Input: dimensioned drawing with shaded views. Units: mm. Origin: part minimum x, y, z. Give positions to 0.01 mm unless a question says otherwise; leave off trailing zeros. Loops run counter-clockwise (first coordinate to the right, second up) from the corner with the lowest first, then second, coordinate; pieces in that order, holes last. Notation, with made-up numbers: (4.25, 8.25) -> (63.25, 8.25) arc R28 cw to (63.25, 28.25) -> close; hole circle Ø3 at (30.25, -5.75). An arc over 180 degrees is marked (long way). Answer as a JSON object with one key per item and string values.
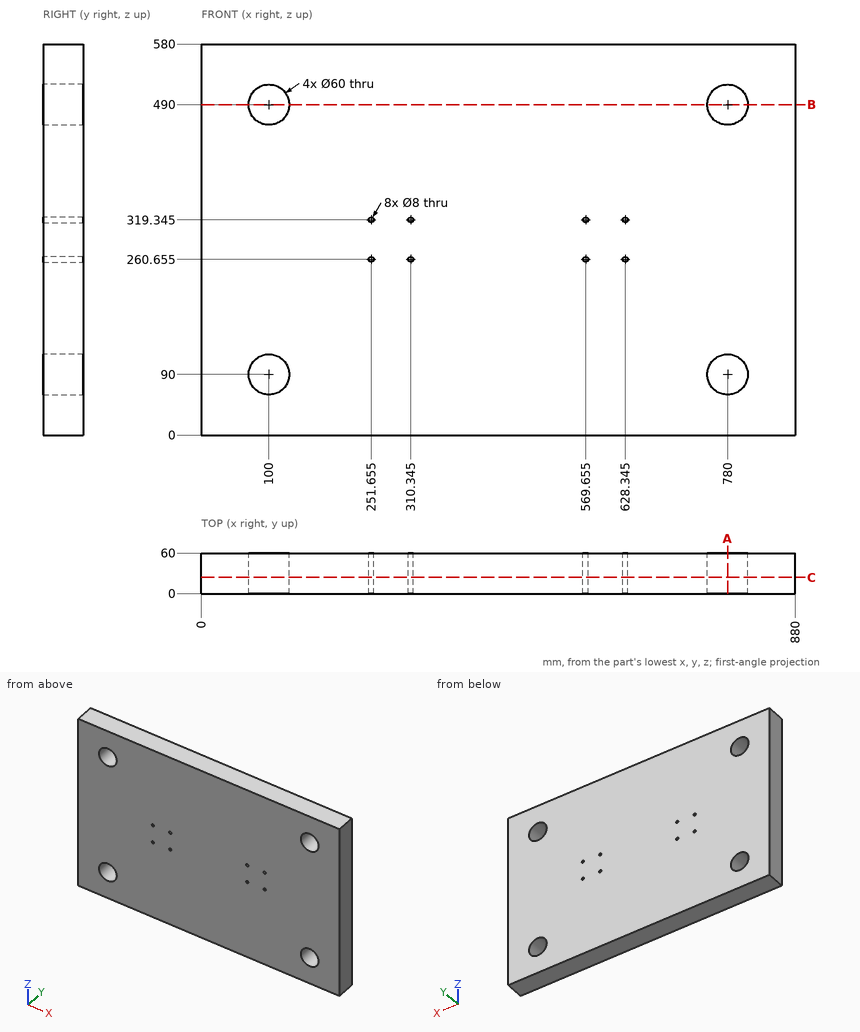
Q1. Ray query, line 1 along X through (y, z) = (57, 261); line 2 along X through (y, z) = (15, 90); line 3 along Z through (x, y) = (254, 46.5). Return the intervals inside material, ascending.
Evaluation:
{"line 1": "x = 0 to 247.67, 255.64 to 306.36, 314.33 to 565.67, 573.64 to 624.36, 632.33 to 880", "line 2": "x = 0 to 70, 130 to 750, 810 to 880", "line 3": "z = 0 to 257.41, 263.9 to 316.1, 322.59 to 580"}
Q2. Section A-A, the plane x = 780. Return the cut outline in (y, z).
Evaluation:
{"outline": "(0, 0) -> (60, 0) -> (60, 60) -> (0, 60) -> close; (0, 120) -> (60, 120) -> (60, 460) -> (0, 460) -> close; (0, 520) -> (60, 520) -> (60, 580) -> (0, 580) -> close"}
Q3. Pin query (flat end, axial travel): pin 1 (7 mm diameter, centred on x = 310.34, z = 319.34, fed in from -Y). Return the tip coordinate at first contact, or that it passes through.
Evaluation:
{"pin 1": "passes through"}
Q4. Section B-B, the plane z = 490. Return the cut outline in (x, y), then the cut area to 3 significant figures.
Evaluation:
{"outline": "(0, 0) -> (70, 0) -> (70, 60) -> (0, 60) -> close; (130, 0) -> (750, 0) -> (750, 60) -> (130, 60) -> close; (810, 0) -> (880, 0) -> (880, 60) -> (810, 60) -> close", "area": "45,600 mm2"}
Q5. Section C-C, the plane y = 24. Give the number of separate pieces and of enclosed holes in the cut face, then the cut area to 3 significant figures.
Evaluation:
{"separate pieces": "1", "enclosed holes": "12", "area": "499,000 mm2"}
